Check sheet for the modelled part. Datum: model origin and axes. Units: mm. Give positions to 0.01 mm unless a question says otherwise; leave off trailing zeros. Loops run counter-clockwise (first coordinate to the right, second up) from the corner with the lowest first, then second, coordinate; pieces in that order, holes last. Notation, with made-up numbers: M -4,-20 L 42,-20 A22 cw 42,-7 Z; hole C 11,89.5 d5. An arc over 180 degrees is marked long. Write each question's results on one line, items separated by ' | '. Start each with the question number.
1. Material ranges on line 1 along Y through (x, z) = (0, 1.4) (3 decimals); line 2 along Y through (x, z) = (17, 1); line 3 along X through (y, z) = (-1.75, 2.05), recorded low to high.
2. Sectioned sample at D-D on y = 5.5. Record the cut outline in (x, z), and give its area (3 significant figures).
3. Go/stop test with flat-tipped pins: pin 1 (2 mm diameter, centred on x = 20.5, y = 6, fed in from -Z); pin 2 (1.9 mm diameter, centred on x = 25.4, y = -8.33, fed in from -Z). Record where each tip stops, or that it passes through.
4. Sectioned sample at C-C on z = 0.85. Give the number of separate pieces and of enclosed holes in the cut face, and give its area (3 significant figures).
5. Sectioned sample at B-B on x = 2. Record the cut outline in (y, z).
6. Sectioned sample at A-A on x = 25.4. Record the cut outline in (y, z) (3 decimals).
```python
from build123d import *

# Parameters (mm, degrees)
SKETCH1_R      = 3.9751
SKETCH1_R_2    = 1.1938
EXTRUDE1_DEPTH = 2.286


with BuildPart() as part:
    # Sketch1 → Extrude1 (new body)
    with BuildSketch(Plane.XY):
        with BuildLine():
            Line((0, 12.2936), (50.8, 12.2936))
            ThreePointArc((50.8, 12.2936), (63.0936, 0), (50.8, -12.2936))
            Line((50.8, -12.2936), (0, -12.2936))
            ThreePointArc((0, -12.2936), (-12.2936, 0), (0, 12.2936))
        make_face()
        Circle(SKETCH1_R, mode=Mode.SUBTRACT)
        with Locations((0, 8.3312)):
            Circle(SKETCH1_R_2, mode=Mode.SUBTRACT)
        with Locations((8.3312, 0)):
            Circle(SKETCH1_R_2, mode=Mode.SUBTRACT)
        with Locations((0, -8.3312)):
            Circle(SKETCH1_R_2, mode=Mode.SUBTRACT)
        with Locations((-8.3312, 0)):
            Circle(SKETCH1_R_2, mode=Mode.SUBTRACT)
        with Locations((17.0688, 0)):
            Circle(SKETCH1_R_2, mode=Mode.SUBTRACT)
        with Locations((33.7312, 0)):
            Circle(SKETCH1_R_2, mode=Mode.SUBTRACT)
        with Locations((25.4, -8.3312)):
            Circle(SKETCH1_R_2, mode=Mode.SUBTRACT)
        with Locations((25.4, 0)):
            Circle(SKETCH1_R, mode=Mode.SUBTRACT)
        with Locations((25.4, 8.3312)):
            Circle(SKETCH1_R_2, mode=Mode.SUBTRACT)
        with Locations((42.4688, 0)):
            Circle(SKETCH1_R_2, mode=Mode.SUBTRACT)
        with Locations((50.8, -8.3312)):
            Circle(SKETCH1_R_2, mode=Mode.SUBTRACT)
        with Locations((59.1312, 0)):
            Circle(SKETCH1_R_2, mode=Mode.SUBTRACT)
        with Locations((50.8, 8.3312)):
            Circle(SKETCH1_R_2, mode=Mode.SUBTRACT)
        with Locations((50.8, 0)):
            Circle(SKETCH1_R, mode=Mode.SUBTRACT)
    extrude(amount=EXTRUDE1_DEPTH)


solid = part.part
```
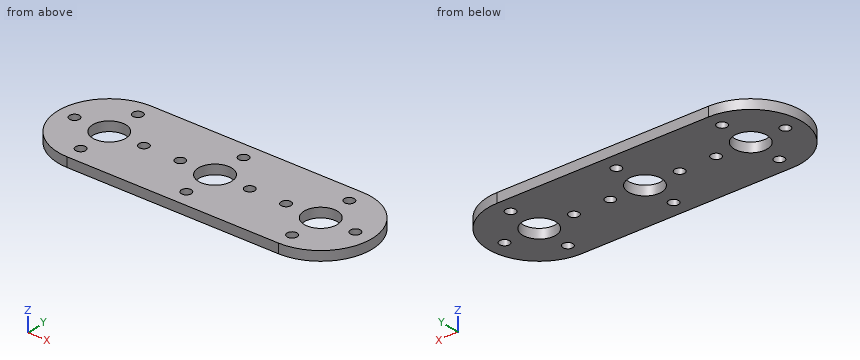
Output values:
1) line 1: -12.294 to -9.525, -7.137 to -3.975, 3.975 to 7.137, 9.525 to 12.294 | line 2: -12.29 to -1.19, 1.19 to 12.29 | line 3: -12.17 to -3.57, 3.57 to 21.83, 28.97 to 47.23, 54.37 to 62.97
2) outline: M -10.99,0 L 61.79,0 L 61.79,2.29 L -10.99,2.29 Z | area: 166 mm2
3) pin 1: z = 0 | pin 2: through
4) separate pieces: 1 | enclosed holes: 15 | area: 1,520 mm2
5) outline: M -12.29,0 L -3.44,0 L -3.44,2.29 L -12.29,2.29 Z; M 3.44,0 L 12.29,0 L 12.29,2.29 L 3.44,2.29 Z
6) outline: M -12.294,0 L -9.525,0 L -9.525,2.286 L -12.294,2.286 Z; M -7.137,0 L -3.975,0 L -3.975,2.286 L -7.137,2.286 Z; M 3.975,0 L 7.137,0 L 7.137,2.286 L 3.975,2.286 Z; M 9.525,0 L 12.294,0 L 12.294,2.286 L 9.525,2.286 Z
